from build123d import *

# Parameters (mm, degrees)
SKETCH1_R           = 2.794
BOSS_EXTRUDE1_DEPTH = 3.937
SKETCH2_R           = 3.81
SKETCH2_R_2         = 2.794
BOSS_EXTRUDE2_DEPTH = 1.27


with BuildPart() as part:
    # Sketch1 → Boss-Extrude1 (new body)
    with BuildSketch(Plane.XY):
        with Locations((7.874, 0)):
            Circle(SKETCH1_R)
        with BuildLine():
            Line((6.35, 0.762), (7.112, 0.762))
            Line((7.112, 0.762), (7.112, 1.524))
            ThreePointArc((7.112, 1.524), (7.874, 2.286), (8.636, 1.524))
            Line((8.636, 1.524), (8.636, 0.762))
            Line((8.636, 0.762), (9.398, 0.762))
            ThreePointArc((9.398, 0.762), (10.16, 0), (9.398, -0.762))
            Line((9.398, -0.762), (8.636, -0.762))
            Line((8.636, -0.762), (8.636, -1.524))
            ThreePointArc((8.636, -1.524), (7.874, -2.286), (7.112, -1.524))
            Line((7.112, -1.524), (7.112, -0.762))
            Line((7.112, -0.762), (6.35, -0.762))
            ThreePointArc((6.35, -0.762), (5.588, 0), (6.35, 0.762))
        make_face(mode=Mode.SUBTRACT)
    boss_extrude1 = extrude(amount=BOSS_EXTRUDE1_DEPTH)

    # Sketch2 → Boss-Extrude2 (add)
    with BuildSketch(Plane(origin=(0, 0, 0), x_dir=(-1, 0, 0), z_dir=(0, 0, -1))):
        with Locations((-7.874, 0)):
            Circle(SKETCH2_R)
        with Locations((-7.874, 0)):
            Circle(SKETCH2_R_2, mode=Mode.SUBTRACT)
    boss_extrude2 = extrude(amount=-BOSS_EXTRUDE2_DEPTH)

    # Mirror1: Boss-Extrude1, Boss-Extrude2 across plane
    add(boss_extrude1.mirror(Plane.XY.offset(3.937)))
    add(boss_extrude2.mirror(Plane.XY.offset(3.937)))


solid = part.part
For this review, take the finished solid that the model builds, in its own axes (mm). A direction names the side the tool comes from. Give positions to 0.01 mm unless a question says otherwise; leave off trailing zeros. Loops run counter-clockwise (first coordinate to the right, second up) from the corner with the lowest first, then second, coordinate; pieces in that order, holes last. Notation, with made-up numbers: (83.25, -21.75) -> (130.25, -21.75) arc R18 cw to (130.25, -11.75) -> close; hole circle Ø1 at (40, -7.75). An arc over 180 degrees is marked (long way). One line per question, with ' | ' between items.
1) Insertion check: pin 1 Ø0.6 at (y, z) = (-1, 1.5) entering from +X; pin 2 Ø1.5 at (y, z) = (1.5, 3.5) entering from -X; pin 3 Ø0.8 at (x, z) = (6.5, 1) entering from -Y. Each pin has a flat end and moves straight along its axis. Give the tip position at first contact, or say it passes through.
Resolved:
pin 1: stops at x = 11.6 | pin 2: stops at x = 5.18 | pin 3: stops at y = -3.68
2) To check wall thickness, follow probe 1 along Z at (x, y) = (10.75, 0.5); probe 2 along X at (y, z) = (-1.25, 4.25); probe 3 along X at (y, z) = (0.5, 0.5). State the ranges of each line that lie inside material, in increasing order.
Resolved:
probe 1: z = 0 to 1.27, 6.6 to 7.87 | probe 2: x = 5.38 to 7.11, 8.64 to 10.37 | probe 3: x = 4.1 to 5.77, 9.97 to 11.65
3) For faces 1 (the cylindrical face through (8.7, -3.72, 0.63)), 2 (the flat face through (9, 3, 6.604)), list the 3-axis set-ups (+Z, -Z, +X, -X, +Y, -Y) from which the entire face can be reached by the end or side of a thin tool; tool diameter is ignored.
Resolved:
face 1: +Z, -Z | face 2: none
4) We need section B-B (y = 0). Write out the cut boundary in (x, z).
Resolved:
outline: (4.06, 0) -> (5.59, 0) -> (5.59, 7.87) -> (4.06, 7.87) -> (4.06, 6.6) -> (5.08, 6.6) -> (5.08, 1.27) -> (4.06, 1.27) -> close; (10.16, 0) -> (11.68, 0) -> (11.68, 1.27) -> (10.67, 1.27) -> (10.67, 6.6) -> (11.68, 6.6) -> (11.68, 7.87) -> (10.16, 7.87) -> close
5) The part is to be moulded in two halves that separate along Z. For faces 3 (the cylindrical face through (8.7, -3.72, 7.25)), 4 (the flat face through (9, 3, 1.27)), 5 (the flat face through (9, -1, 7.874)), say which applies: +Z half, -Z half, draft (parallel to the pull), parting line (faces both ways), or undercut.
Resolved:
face 3: draft | face 4: undercut | face 5: +Z half
6) We need section A-A (z = 2.5). Write out the cut boundary in (x, y).
Resolved:
outline: circle Ø5.59 at (7.87, 0); hole (6.35, -0.76) -> (7.11, -0.76) -> (7.11, -1.52) arc R0.76 ccw to (8.64, -1.52) -> (8.64, -0.76) -> (9.4, -0.76) arc R0.76 ccw to (9.4, 0.76) -> (8.64, 0.76) -> (8.64, 1.52) arc R0.76 ccw to (7.11, 1.52) -> (7.11, 0.76) -> (6.35, 0.76) arc R0.76 ccw to start
7) We need section C-C (x = 6.5). Write out the cut boundary in (y, z).
Resolved:
outline: (-3.55, 0) -> (-0.76, 0) -> (-0.76, 7.87) -> (-3.55, 7.87) -> (-3.55, 6.6) -> (-2.43, 6.6) -> (-2.43, 1.27) -> (-3.55, 1.27) -> close; (0.76, 0) -> (3.55, 0) -> (3.55, 1.27) -> (2.43, 1.27) -> (2.43, 6.6) -> (3.55, 6.6) -> (3.55, 7.87) -> (0.76, 7.87) -> close
8) We need section D-D (z = 6.75). Write out the cut boundary in (x, y).
Resolved:
outline: circle Ø7.62 at (7.87, 0); hole (6.35, -0.76) -> (7.11, -0.76) -> (7.11, -1.52) arc R0.76 ccw to (8.64, -1.52) -> (8.64, -0.76) -> (9.4, -0.76) arc R0.76 ccw to (9.4, 0.76) -> (8.64, 0.76) -> (8.64, 1.52) arc R0.76 ccw to (7.11, 1.52) -> (7.11, 0.76) -> (6.35, 0.76) arc R0.76 ccw to start
